Design review of the part built by this model. Coordinates are the model's own, in mm. A direction names the side the tool comes from. Coordinates: 2 decimals unless noted, no trailing zeros. Loops run counter-clockwise (first coordinate to the right, second up) from the corner with the lowest first, then second, coordinate; pieces in that order, holes last. Notation, with made-up numbers: (17.5, 27.25) - (47.5, 27.25) arc R17 ccw to (47.5, 40.25) - close; hole circle Ø9 at (87, 69.5). An arc over 180 degrees is marked (long way). Return JSON: item names as keys, results as strings. Group by question number.
from build123d import *

# Parameters (mm, degrees)
F0_W     = 200
F0_H     = 150
F1_DEPTH = 19
F2_W     = 20
F2_H     = 20
F2_H_2   = 110
F3_DEPTH = 19
F4_R     = 4.75
F5_DEPTH = 150
F7_DEPTH = 19


with BuildPart() as f1:
    # F0 (on Top) → F1 (new body)
    with BuildSketch(Plane.XY):
        with Locations((100, 75)):
            Rectangle(F0_W, F0_H)
    extrude(amount=F1_DEPTH)

    # F2 (on face) → F3 (cut)
    with BuildSketch(Plane.XY.offset(19)):
        with Locations((10, 140)):
            Rectangle(F2_W, F2_H)
        with Locations((10, 10)):
            Rectangle(F2_W, F2_H)
        with Locations((190, 75)):
            Rectangle(F2_W, F2_H_2)
    extrude(amount=-F3_DEPTH, mode=Mode.SUBTRACT)

    # F4 (on face) → F5 (cut)
    with BuildSketch(Plane(origin=(0, 150, 0), x_dir=(-1, 0, 0), z_dir=(0, 1, 0))):
        with Locations((-12, 10)):
            Circle(F4_R)
        with Locations((-188, 10)):
            Circle(F4_R)
    extrude(amount=-F5_DEPTH, mode=Mode.SUBTRACT)

    # F6 (on face) → F7 (cut)
    with BuildSketch(Plane.XY.offset(19)):
        with BuildLine():
            Line((170, 147), (170, 150))
            Line((170, 150), (156, 150))
            Line((156, 150), (156, 147))
            ThreePointArc((156, 147), (153.366454, 140.237208), (146.852929, 137.036441))
            Line((146.852929, 137.036441), (51.95297, 128.912542))
            ThreePointArc((51.95297, 128.912542), (30, 105), (51.95297, 81.087458))
            Line((51.95297, 81.087458), (146.852929, 72.963559))
            ThreePointArc((146.852929, 72.963559), (156, 63), (146.852929, 53.036441))
            Line((146.852929, 53.036441), (51.95297, 44.912542))
            ThreePointArc((51.95297, 44.912542), (38.08635, 38.965404), (30.509258, 25.917827))
            Line((30.509258, 25.917827), (28.190972, 14.844185))
            ThreePointArc((28.190972, 14.844185), (38.748466, 4.171474), (44.441179, 18.062496))
            ThreePointArc((44.441179, 18.062496), (45.71082, 26.593702), (53.147071, 30.963559))
            Line((53.147071, 30.963559), (148.04703, 39.087458))
            ThreePointArc((148.04703, 39.087458), (170, 63), (148.04703, 86.912542))
            Line((148.04703, 86.912542), (53.147071, 95.036441))
            ThreePointArc((53.147071, 95.036441), (44, 105), (53.147071, 114.963559))
            Line((53.147071, 114.963559), (148.04703, 123.087458))
            ThreePointArc((148.04703, 123.087458), (163.67949, 130.769299), (170, 147))
        make_face()
    extrude(amount=-F7_DEPTH, mode=Mode.SUBTRACT)


solid = f1.part
Item 1: For faces 1 (the face through (194, 130, 10)), 2 (the face through (20, 140, 10)), 3 (the face through (156, 63, 10)), list the 3-axis set-ups (+Z, -Z, +X, -X, +Y, -Y) from which the entire face can be reached by the end or side of a thin tool; tool diameter is ignored.
Item 2: Add section A-A (y = 57). State the section outline as (x, z) points.
Item 3: Add section B-B (x = 12). State the section outline as (y, z) points, then the cut area to 4 significant figures.
Item 4: Draft analysis for pull direction X (two halves, no side actions). For faces 4 (the face through (29.366, 20.459, 9.633)), 5 (the face through (200, 140, 9)), 6 (the face through (194, 20, 10)), state which applies: pulls with the +X half, pulls with the -X half, needs draft (parallel to the pull), parting line crosses it, or undercut.
Item 5: To check wall thickness, follow line 1 (X direction, y = 13.5, z = 15.75); line 2 (Z direction, x = 188, y = 15.75); line 3 (X direction, y = 96.5, z = 14). State the ranges of each line that lie inside material, in increasing order. Write a range as from..to.
Item 6: Add section D-D (y = 78.5). State the section outline as (x, z) points, then the cut area to 3 significant figures.
Item 7: Add section C-C (x = 188). State the section outline as (y, z) points, then the cut area to 3 significant figures.
Item 8: For P1, Ø9.5, axis at x = 12, z = 14, coming from the +Y side; P2, Ø4, axis at y = 132.5, z = 2.5, coming from the -X side; P3, Ø1, axis at y = 98, z = 9.5, coming from the -X side; P4, Ø5.5, axis at y = 51, z = 13.5, coming from the +X side, all flat-tipped, find the tip position at first contact; note any pin that passes through.
Answers below:
{
 "1": {"face 1": "+Z, -Z, +X", "face 2": "+Z, -Z, -X, +Y", "face 3": "+Z, -Z"},
 "2": {"outline": "(0, 0) - (154, 0) - (154, 19) - (0, 19) - close; (169.24, 0) - (180, 0) - (180, 19) - (169.24, 19) - close; hole circle Ø9.5 at (12, 10)"},
 "3": {"outline": "(20, 0) - (130, 0) - (130, 5.25) - (20, 5.25) - close; (20, 14.75) - (130, 14.75) - (130, 19) - (20, 19) - close", "area": "1,045 mm^2"},
 "4": {"face 4": "undercut", "face 5": "pulls with the +X half", "face 6": "needs draft"},
 "5": {"line 1": "x = 20..28.01, 45.99..200", "line 2": "z = 0..5.25, 14.75..19", "line 3": "x = 0..9.44, 14.56..31.56, 48.73..180"},
 "6": {"outline": "(0, 0) - (82.18, 0) - (82.18, 19) - (0, 19) - close; (164.32, 0) - (180, 0) - (180, 19) - (164.32, 19) - close; hole circle Ø9.5 at (12, 10)", "area": "1,790 mm^2"},
 "7": {"outline": "(0, 0) - (20, 0) - (20, 5.25) - (0, 5.25) - close; (0, 14.75) - (20, 14.75) - (20, 19) - (0, 19) - close; (130, 0) - (150, 0) - (150, 5.25) - (130, 5.25) - close; (130, 14.75) - (150, 14.75) - (150, 19) - (130, 19) - close", "area": "380 mm^2"},
 "8": {"P1": "stops at y = 130", "P2": "stops at x = 20", "P3": "stops at x = 0", "P4": "stops at x = 180"}
}
